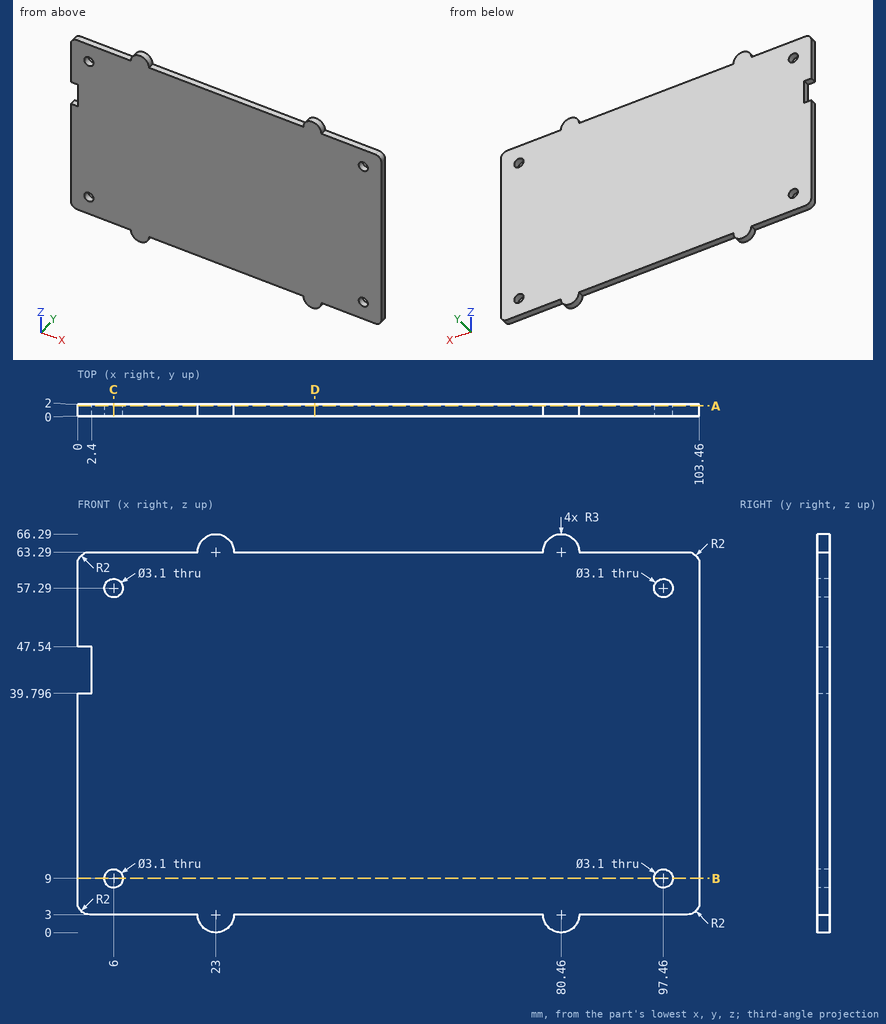
Check sheet for the drawn part. Datum: minimum x, y, z corner. Units: mm. Give positions to 0.01 mm unless a question says otherwise; leave off trailing zeros. Write each loop counter-clockwise with the first axis right and the second up, starting at its lowest first coordinate (ties: lowest second). Pieces come first, ordered by that corner, then holes.
(1) Cross-section at B-B (z = 9). Enter the section's corners in (x, y).
(2) Cross-section at A-A (y = 1.7). Enter the section's corners in (x, z).
(3) Material ranges on line 1 (X direction, y = 1.25, z = 9); line 2 (Z direction, x = 97.46, y = 1); line 3 (Z direction, x = 98, y = 0.7), recorded low to high.
(4) Cross-section at D-D (x = 39.5). Enter the section's corners in (y, z).
(5) Gauge pin test, flat ends, axial feed: pin 1 (3 mm diameter, centred on x = 6, z = 9, fed in from -Y); pin 2 (3.5 mm diameter, centred on x = 97.46, z = 9, fed in from +Y); pin 3 (1 mm diameter, centred on x = 12.5, y = 1.5, fed in from +Z); pin 4 (1 mm diameter, centred on x = 43.5, y = 1, fed in from -Z). Record the tip position at first contact, or that the pin passes through.
(6) Cross-section at C-C (x = 6). Enter the section's corners in (y, z).
Worked out:
1. outline: (0, 0) - (4.45, 0) - (4.45, 2) - (0, 2) - close; (7.55, 0) - (95.91, 0) - (95.91, 2) - (7.55, 2) - close; (99.01, 0) - (103.46, 0) - (103.46, 2) - (99.01, 2) - close
2. outline: (0, 5) arc R2 ccw to (2, 3) - (20, 3) arc R3 ccw to (26, 3) - (77.46, 3) arc R3 ccw to (83.46, 3) - (101.46, 3) arc R2 ccw to (103.46, 5) - (103.46, 61.29) arc R2 ccw to (101.46, 63.29) - (83.46, 63.29) arc R3 ccw to (77.46, 63.29) - (26, 63.29) arc R3 ccw to (20, 63.29) - (2, 63.29) arc R2 ccw to (0, 61.29) - (0, 47.54) - (2.4, 47.54) - (2.4, 39.8) - (0, 39.8) - close; hole circle Ø3.1 at (6, 9); hole circle Ø3.1 at (6, 57.29); hole circle Ø3.1 at (97.46, 9); hole circle Ø3.1 at (97.46, 57.29)
3. line 1: x = 0 to 4.45, 7.55 to 95.91, 99.01 to 103.46
3. line 2: z = 3 to 7.45, 10.55 to 55.74, 58.84 to 63.29
3. line 3: z = 3 to 7.55, 10.45 to 55.84, 58.74 to 63.29
4. outline: (0, 3) - (2, 3) - (2, 63.29) - (0, 63.29) - close
5. pin 1: passes through
5. pin 2: stops at y = 2
5. pin 3: stops at z = 63.29
5. pin 4: stops at z = 3
6. outline: (0, 3) - (2, 3) - (2, 7.45) - (0, 7.45) - close; (0, 10.55) - (2, 10.55) - (2, 55.74) - (0, 55.74) - close; (0, 58.84) - (2, 58.84) - (2, 63.29) - (0, 63.29) - close
